```python
from build123d import *

# Parameters (mm, degrees)
SKETCH1_R                   = 13.21
SKETCH1_R_2                 = 2.585
BOSS_EXTRUDE1_DEPTH         = 20
CHAMFER1_SIZE               = 1.2
BOSS_EXTRUDE5_START         = 40
SKETCH7_R                   = 13.21
SKETCH7_R_2                 = 3.785
BOSS_EXTRUDE5_DEPTH         = 40
CUT_EXTRUDE3_DEPTH          = 0.7
CUT_EXTRUDE3_DEPTH_BACK     = 0.7
SKETCH8_W                   = 13.21
SKETCH8_H                   = 35.8
SKETCH11_W                  = 13.21
SKETCH11_H                  = 35.8
CUT_EXTRUDE5_DEPTH          = 2.5
CUT_EXTRUDE6_DEPTH          = 45.362058113
CUT_EXTRUDE6_DEPTH_BACK     = 45.362058113
SKETCH12_R                  = 1.2
SKETCH13_R                  = 2.5
CUT_EXTRUDE7_DEPTH          = 47.174584074
SKETCH15_R                  = 1.8
BOSS_EXTRUDE6_DEPTH         = 5
BOSS_EXTRUDE7_REACH         = 61.49
CIRPATTERN2_COUNT           = 4
CIRPATTERN2_COPY_1_SKETCH_R = 1.8
CIRPATTERN2_COPY_1_DEPTH    = 5
CIRPATTERN2_COPY_2_SKETCH_R = 1.8
CIRPATTERN2_COPY_2_DEPTH    = 5
CIRPATTERN2_COPY_3_SKETCH_R = 1.8
CIRPATTERN2_COPY_3_DEPTH    = 5
CHAMFER2_SIZE               = 15
CHAMFER2_SIZE2              = 6.994614872


with BuildPart() as part:
    # Sketch1 → Boss-Extrude1 (new body)
    with BuildSketch(Plane(origin=(0, 0, 0), x_dir=(1, 0, 0), z_dir=(0, 1, 0))):
        with Locations(Location((0, 0, 0), (0, 0, 270))):
            Circle(SKETCH1_R)
        with Locations(Location((0, 0, 0), (0, 0, 270))):
            Circle(SKETCH1_R_2, mode=Mode.SUBTRACT)
    extrude(amount=BOSS_EXTRUDE1_DEPTH)

    # Chamfer1
    chamfer1_edges = [part.edges().sort_by_distance(p)[0] for p in [
        (0, 0, -2.585),
    ]]
    chamfer(chamfer1_edges, length=CHAMFER1_SIZE)

    # Sketch7 → Boss-Extrude5 (add)
    with BuildSketch(Plane.XZ.offset(BOSS_EXTRUDE5_START)):
        with Locations(Location((0, 0, 0), (0, 0, 270))):
            Circle(SKETCH7_R)
        with Locations(Location((0, 0, 0), (0, 0, 270))):
            Circle(SKETCH7_R_2, mode=Mode.SUBTRACT)
    extrude(amount=-BOSS_EXTRUDE5_DEPTH)

    # Sketch8 → Cut-Extrude3 (cut, two sides: drawn at the far end of the back side and taken through both)
    with BuildSketch(Plane(origin=(0, 0, 0), x_dir=(0, 0, -1), z_dir=(1, 0, 0)).offset(-CUT_EXTRUDE3_DEPTH_BACK)):
        with Locations((-6.605, -22.1)):
            Rectangle(SKETCH8_W, SKETCH8_H)
    extrude(amount=CUT_EXTRUDE3_DEPTH + CUT_EXTRUDE3_DEPTH_BACK, mode=Mode.SUBTRACT)

    # Sketch11 → Cut-Extrude5 (cut, symmetric)
    with BuildSketch(Plane(origin=(0, 0, 0), x_dir=(0, 0, -1), z_dir=(1, 0, 0))):
        with Locations((6.605, -22.1)):
            Rectangle(SKETCH11_W, SKETCH11_H)
    extrude(amount=CUT_EXTRUDE5_DEPTH, both=True, mode=Mode.SUBTRACT)

    # Sketch12 → Cut-Extrude6 (cut, two sides: drawn at the far end of the back side and taken through both)
    with BuildSketch(Plane.ZY.offset(-0.7).offset(-CUT_EXTRUDE6_DEPTH_BACK)):
        with Locations((10.21, -8.2)):
            Circle(SKETCH12_R)
    extrude(amount=CUT_EXTRUDE6_DEPTH + CUT_EXTRUDE6_DEPTH_BACK, mode=Mode.SUBTRACT)

    # Sketch13 → Cut-Extrude7 (cut, through all)
    with BuildSketch(Plane.ZY.offset(-5.7)):
        with Locations((10.21, -8.2)):
            Circle(SKETCH13_R)
    cut_extrude7 = extrude(amount=-CUT_EXTRUDE7_DEPTH, mode=Mode.SUBTRACT)

    # Mirror2: Cut-Extrude7 across plane
    add(cut_extrude7.mirror(Plane(origin=(0, 0, 0), x_dir=(0, 0, 1), z_dir=(1, 0, 0))), mode=Mode.SUBTRACT)

    # Sketch15 → Boss-Extrude6 (add)
    with BuildSketch(Plane(origin=(-1.060660172, 0, -1.060660172), x_dir=(-0.7071067811865488, -3.372135297382167e-15, 0.7071067811865462), z_dir=(-0.7071067811865462, 3.3721352973821793e-15, -0.7071067811865488))):
        Polygon((-22.70423895, -23.81017386), (-11.21, -23.81017386), (-11.21, -35.211035784), (-11.21, -40), (-15.990174244, -46.657077484), (-29.831605047, -40.876524454), align=None)
        with Locations((-19.21, -29.81017386)):
            Circle(SKETCH15_R, mode=Mode.SUBTRACT)
        with Locations((-19.21, -38.81017386)):
            Circle(SKETCH15_R, mode=Mode.SUBTRACT)
    boss_extrude6 = extrude(amount=BOSS_EXTRUDE6_DEPTH)

    # Mirror3: Boss-Extrude6 across plane
    add(boss_extrude6.mirror(Plane(origin=(0, 0, 0), x_dir=(-0.7071067811865488, 3.3721352973821916e-15, 0.7071067811865464), z_dir=(0.7071067811865462, -3.3721352973821793e-15, 0.7071067811865488))))

    # Boss-Extrude7: up to this face of the body (flat: up to its plane)
    boss_extrude7_end = Plane(part.part.faces().sort_by_distance((18.066702505, -34.728946199, -8.87431435))[0])
    # Sketch16 → Boss-Extrude7 (add, up to the picked face)
    with BuildSketch(Plane(origin=(-4.596194078, 0, -4.596194078), x_dir=(-0.7071067811865486, -3.1363800445660566e-15, 0.7071067811865465), z_dir=(-0.7071067811865465, 3.1363800445660664e-15, -0.7071067811865486)), mode=Mode.PRIVATE) as boss_extrude7_sk1:
        with BuildLine():
            Line((-11.500178259, -23.81017386), (-22.70423895, -23.81017386))
            ThreePointArc((-22.70423895, -23.81017386), (-18.231146382, -18.383887076), (-11.500178259, -16.347416226))
            Line((-11.500178259, -16.347416226), (-11.500178259, -23.81017386))
        make_face()
    boss_extrude7_tool1 = split(extrude(boss_extrude7_sk1.sketch, amount=-BOSS_EXTRUDE7_REACH, mode=Mode.PRIVATE), bisect_by=boss_extrude7_end, keep=Keep.BOTH, mode=Mode.PRIVATE)
    boss_extrude7 = boss_extrude7_tool1.solids().sort_by(Axis((6.682248, -20.729124, -15.874636), (0.7071067811865465, -3.1363800445660664e-15, 0.7071067811865486)))[0]
    add(boss_extrude7)

    # CirPattern2: Boss-Extrude6, Boss-Extrude7 ×4 about axis
    cirpattern2_axis = Axis((0, 0, 0), (0, 1, 0))
    add([boss_extrude6.rotate(cirpattern2_axis, i * 360 / CIRPATTERN2_COUNT) for i in range(1, CIRPATTERN2_COUNT)])
    add([boss_extrude7.rotate(cirpattern2_axis, i * 360 / CIRPATTERN2_COUNT) for i in range(1, CIRPATTERN2_COUNT)])

    # CirPattern2 copy 1 sketch → CirPattern2 copy 1 (add)
    with BuildSketch(Plane(origin=(1.060660172, 0, -1.060660172), x_dir=(0.7071067811865462, -3.372135297382167e-15, 0.7071067811865489), z_dir=(0.7071067811865488, -3.3721352973821793e-15, -0.7071067811865461))):
        Polygon((-22.70423895, 23.81017386), (-11.21, 23.81017386), (-11.21, 35.211035784), (-11.21, 40), (-15.990174244, 46.657077484), (-29.831605047, 40.876524454), align=None)
        with Locations((-19.21, 29.81017386)):
            Circle(CIRPATTERN2_COPY_1_SKETCH_R, mode=Mode.SUBTRACT)
        with Locations((-19.21, 38.81017386)):
            Circle(CIRPATTERN2_COPY_1_SKETCH_R, mode=Mode.SUBTRACT)
    extrude(amount=CIRPATTERN2_COPY_1_DEPTH)

    # CirPattern2 copy 2 sketch → CirPattern2 copy 2 (add)
    with BuildSketch(Plane(origin=(-1.060660172, 0, -1.060660172), x_dir=(0.7071067811865489, -3.372135297382167e-15, -0.7071067811865462), z_dir=(-0.7071067811865461, -3.3721352973821793e-15, -0.7071067811865488))):
        Polygon((-22.70423895, 23.81017386), (-11.21, 23.81017386), (-11.21, 35.211035784), (-11.21, 40), (-15.990174244, 46.657077484), (-29.831605047, 40.876524454), align=None)
        with Locations((-19.21, 29.81017386)):
            Circle(CIRPATTERN2_COPY_2_SKETCH_R, mode=Mode.SUBTRACT)
        with Locations((-19.21, 38.81017386)):
            Circle(CIRPATTERN2_COPY_2_SKETCH_R, mode=Mode.SUBTRACT)
    extrude(amount=CIRPATTERN2_COPY_2_DEPTH)

    # CirPattern2 copy 3 sketch → CirPattern2 copy 3 (add)
    with BuildSketch(Plane(origin=(-1.060660172, 0, 1.060660172), x_dir=(-0.7071067811865461, -3.372135297382167e-15, -0.707106781186549), z_dir=(-0.7071067811865489, -3.3721352973821793e-15, 0.707106781186546))):
        Polygon((-22.70423895, 23.81017386), (-11.21, 23.81017386), (-11.21, 35.211035784), (-11.21, 40), (-15.990174244, 46.657077484), (-29.831605047, 40.876524454), align=None)
        with Locations((-19.21, 29.81017386)):
            Circle(CIRPATTERN2_COPY_3_SKETCH_R, mode=Mode.SUBTRACT)
        with Locations((-19.21, 38.81017386)):
            Circle(CIRPATTERN2_COPY_3_SKETCH_R, mode=Mode.SUBTRACT)
    extrude(amount=CIRPATTERN2_COPY_3_DEPTH)

    # Chamfer2
    chamfer2_edges = [part.edges().sort_by_distance(p)[0] for p in [
        (0, 20, -13.21),
    ]]
    chamfer2_side = [part.faces().sort_by_distance(p)[0] for p in [
        (0, 10, -13.21),
    ]]
    chamfer(chamfer2_edges, length=CHAMFER2_SIZE, length2=CHAMFER2_SIZE2, reference=chamfer2_side[0])


solid = part.part
```
Model file for the job. Use its own axes, mm. A direction names the side the tool comes from. Give positions to 0.01 mm unless a question says otherwise; leave off trailing zeros. Write each loop counter-clockwise with the first axis right and the second up, starting at its lowest first coordinate (ties: lowest second). Pieces come first, ordered by that corner, then holes. Notation, with made-up numbers: M 25.25,2 L 58.25,2 A19 ccw 58.25,10 Z; hole C -20.75,-2 d6. An arc over 180 degrees is marked long. Use a Markdown table: item, result.
1) Pin check, flat tips, straight feed: pin 1 (5.5 mm diameter, centred on x = 0, z = -9, fed in from -Y); pin 2 (4.5 mm diameter, centred on y = -8.2, z = 10.21, fed in from -X); pin 3 (6.5 mm diameter, centred on y = -8.2, z = 10.21, fed in from +X); pin 4 (4.5 mm diameter, centred on x = 0, z = 0, fed in from -Y). Stop position of each tip, or through.
Responses:
| item | result |
|---|---|
| pin 1 | stops at y = -40 |
| pin 2 | stops at x = -5.7 |
| pin 3 | stops at x = 11.23 |
| pin 4 | passes through |
2) Pull direction X, two halves, no side cores. Call faces 1 (the cylindrical face through (2.18, 10.47, 1.39)), 2 (the conical face through (-4.93, 15.94, -6.44)), 3 (the cylindrical face through (-13.01, -18.44, -12.89)): +X half, -X half, draft (parallel to the pull), parting line (faces both ways), or undercut.
Responses:
| item | result |
|---|---|
| face 1 | undercut |
| face 2 | parting line |
| face 3 | -X half |
3) Drill centre lines: line 1 (X direction, y = -40, z = -19); line 2 (Z direction, x = -2.95, y = -8.2); line 3 (Z direction, x = 3, y = -8). Where is each one in solid material? Low to high. Write a range as from..to.
Responses:
| item | result |
|---|---|
| line 1 | x = -22.67..-21.12, -16.88..-10.08, 10.08..16.88, 21.12..22.67 |
| line 2 | z = -12.88..-2.37, 2.37..9.01, 11.41..12.88 |
| line 3 | z = -12.86..-2.31, 2.31..9.03, 11.39..12.86 |
4) Tool access for faces 4 (the cylindrical face through (-7.62, -8.12, 7.71)), 5 (the flat face through (21.41, -32.46, -15.81)), 6 (the flat face through (6.789, -43.282, 12.397)): list every direction of +Z, -Z, +X, -X, +Y, -Y with a clear straight run to the whole face (end or side of a thin tool).
Responses:
| item | result |
|---|---|
| face 4 | -X |
| face 5 | -Z, +X, +Y |
| face 6 | -Y |
5) Cut at B-B (z = 0). List the corners of the cut face in (x, y) (3 decimals).
Responses:
| item | result |
|---|---|
| outline | M -13.21,-40 L -3.785,-40 L -3.785,0 L -2.585,1.2 L -2.585,20 L -6.215,20 L -13.21,5 Z; M 2.585,1.2 L 3.785,0 L 3.785,-40 L 13.21,-40 L 13.21,5 L 6.215,20 L 2.585,20 Z |
6) Cut at A-A (y = -8.2). List the corners of the cut face in (x, z) (3 decimals), and give its area (3 significant figures).
Responses:
| item | result |
|---|---|
| outline | M -10.727,7.71 A13.21 ccw -2.5,-12.971 L -2.5,-2.842 A3.785 cw -0.7,3.72 L -0.7,9.01 L -5.7,9.01 L -5.7,7.71 Z; M -5.7,11.41 L -0.7,11.41 L -0.7,13.191 A13.21 ccw -5.7,11.917 Z; M 0.7,3.72 A3.785 cw 2.5,-2.842 L 2.5,-12.971 A13.21 ccw 10.727,7.71 L 5.7,7.71 L 5.7,9.01 L 0.7,9.01 Z; M 0.7,11.41 L 5.7,11.41 L 5.7,11.917 A13.21 ccw 0.7,13.191 Z |
| area | 393 mm2 |
